from build123d import *

# Parameters (mm, degrees)
F0_W     = 52
F0_H     = 52
F0_R     = 20
F1_DEPTH = 3
F0_R_2   = 17.5
F0_R_3   = 2.5
F2_DEPTH = 25.4
F3_DEPTH = 1.55
F4_R     = 12.5
F5_R     = 1.5
F6_R     = 3
F7_W     = 5
F7_H     = 1.5
F8_DEPTH = 25.4
F9_R     = 1


with BuildPart() as f1:
    # F0 (on Top) → F1 (new body)
    with BuildSketch(Plane.XY):
        Rectangle(F0_W, F0_H)
        Circle(F0_R, mode=Mode.SUBTRACT)
    extrude(amount=F1_DEPTH)



with BuildPart() as f1b:
    # F0 (on Top) → F1, piece 2 (new body)
    with BuildSketch(Plane.XY):
        Circle(F0_R_2)
        Circle(F0_R_3, mode=Mode.SUBTRACT)
    extrude(amount=F1_DEPTH)


with BuildPart() as f1_1:
    add(f1.part)

    add(f1b.part)  # F2 merges F1b
    # F0 (on Top) → F2 (join)
    with BuildSketch(Plane.XY):
        Circle(F0_R)
        Circle(F0_R_2, mode=Mode.SUBTRACT)
    extrude(amount=F2_DEPTH)

    # F0 (on Top) → F3 (cut)
    with BuildSketch(Plane.XY):
        Circle(F0_R_2)
        Circle(F0_R_3, mode=Mode.SUBTRACT)
    extrude(amount=F3_DEPTH, mode=Mode.SUBTRACT)

    # F4
    f4_edges = [f1_1.edges().sort_by_distance(p)[0] for p in [
        (-26, 26, 1.5),
        (26, 26, 1.5),
        (26, -26, 1.5),
        (-26, -26, 1.5),
    ]]
    fillet(f4_edges, radius=F4_R)

    # F5
    f5_edges = [f1_1.edges().sort_by_distance(p)[0] for p in [
        (-20, 0, 25.4),
        (0, -26, 3),
    ]]
    fillet(f5_edges, radius=F5_R)

    # F6
    f6_edges = [f1_1.edges().sort_by_distance(p)[0] for p in [
        (-20, 0, 3),
    ]]
    fillet(f6_edges, radius=F6_R)

    # F7 (on face) → F8 (cut)
    with BuildSketch(Plane.XZ.offset(26)):
        with Locations((0, 0.75)):
            Rectangle(F7_W, F7_H)
    extrude(amount=-F8_DEPTH, mode=Mode.SUBTRACT)

    # F9
    f9_edges = [f1_1.edges().sort_by_distance(p)[0] for p in [
        (-2.5, -21.660254, 1.5),
        (2.5, -21.660254, 1.5),
    ]]
    fillet(f9_edges, radius=F9_R)


solid = f1_1.part
Geometry check sheet. Reference: the model listing, model coordinates, mm. A direction names the side the tool comes from. Give positions to 0.01 mm unless a question says otherwise; leave off trailing zeros. Order: outer loops, then holes, each group sorted by start corner. A loop starts at its lowest first (then second) coordinate and runs counter-clockwise, first axis right, second up.
1) Cross-section at A-A (x = 0). Record the boundary of the cut face in (y, z).
Results are:
outline: (-26, 1.5) - (-17.5, 1.5) - (-17.5, 1.55) - (-2.5, 1.55) - (-2.5, 3) - (-17.5, 3) - (-17.5, 25.4) - (-18.5, 25.4) arc R1.5 ccw to (-20, 23.9) - (-20, 6) arc R3 cw to (-23, 3) - (-24.5, 3) arc R1.5 ccw to start; (2.5, 1.55) - (17.5, 1.55) - (17.5, 0) - (26, 0) - (26, 1.5) arc R1.5 ccw to (24.5, 3) - (23, 3) arc R3 cw to (20, 6) - (20, 23.9) arc R1.5 ccw to (18.5, 25.4) - (17.5, 25.4) - (17.5, 3) - (2.5, 3) - close
2) Cross-section at B-B (y = 0). Record the boundary of the cut face in (x, z), then the cut area to 3 significant figures.
Results are:
outline: (-26, 0) - (-17.5, 0) - (-17.5, 1.55) - (-2.5, 1.55) - (-2.5, 3) - (-17.5, 3) - (-17.5, 25.4) - (-18.5, 25.4) arc R1.5 ccw to (-20, 23.9) - (-20, 6) arc R3 cw to (-23, 3) - (-24.5, 3) arc R1.5 ccw to (-26, 1.5) - close; (2.5, 1.55) - (17.5, 1.55) - (17.5, 0) - (26, 0) - (26, 1.5) arc R1.5 ccw to (24.5, 3) - (23, 3) arc R3 cw to (20, 6) - (20, 23.9) arc R1.5 ccw to (18.5, 25.4) - (17.5, 25.4) - (17.5, 3) - (2.5, 3) - close
area: 208 mm2
3) Gauge pin test, flat ends, axial feed: pin 1 (10.5 mm diameter, centred on x = 8, y = 5, fed in from -Z); pin 2 (3 mm diameter, centred on x = 0, y = 0, fed in from -Z); pin 3 (5 mm diameter, centred on y = -12.5, z = 4.5, fed in from +X); pin 4 (5 mm diameter, centred on y = 14.5, z = 15.5, fed in from +X). Record the tip position at first contact, or that the pin passes through.
Results are:
pin 1: stops at z = 1.55
pin 2: passes through
pin 3: stops at x = 25.91
pin 4: stops at x = 16
4) Draft check along Y on faces 4 (the cylindrical face through (-0.54, -2.44, 2.26)), 5 (the cylindrical face through (-0.19, 25.55, 2.57)), 6 (the flat face through (26, 0, 1)). Enter one of: released by +Y, released by -Y, zero draft, split by the parting line, or undercut.
Results are:
face 4: undercut
face 5: released by +Y
face 6: zero draft
5) Material ranges on probe 1 along Y at (x, z) = (0, 18.75); probe 2 along X at (y, z) = (0, 0.8); probe 3 along X at (y, z) = (-3, 3.25), recorded low to high.
Results are:
probe 1: y = -20 to -17.5, 17.5 to 20
probe 2: x = -26 to -17.5, 17.5 to 26
probe 3: x = -21.59 to -17.24, 17.24 to 21.59
6) Tool access check on faces 1 (the flat face through (0, -22, 1.5)), 2 (the flat face through (0, -4, 3)), 3 (the flat face through (0, -4, 1.55)). Record the directions out of +Z, -Z, +X, -X, +Y, -Y that give a thin tool (end or side, any length) a straight path to the whole face; none if there is none.
Results are:
face 1: -Z, -Y
face 2: +Z
face 3: -Z
7) Cross-section at C-C (z = 18.25). Record the boundary of the cut face in (x, y).
Results are:
outline: circle Ø40 at (0, 0); hole circle Ø35 at (0, 0)
